Read the model definition and answer for the solid it produces. Units are mm, in the model's axes. A direction names the side the tool comes from. Coordinates: 2 decimals unless noted, no trailing zeros. Order: outer loops, then holes, each group sorted by start corner. A loop starts at its lowest first (then second) coordinate and runs counter-clockwise, first axis right, second up. Notation, with made-up numbers: (-39.5, 27.25) - (-23.5, 27.25) arc R21 ccw to (-23.5, 37.25) - close; hole circle Ø5 at (87.5, 31.25). An arc over 180 degrees is marked (long way). Answer as a JSON object with one key per item and string values. Group by question number.
from build123d import *

# Parameters (mm, degrees)
SKETCH1_W           = 12
SKETCH1_H           = 22
BOSS_EXTRUDE1_DEPTH = 23
SKETCH3_W           = 12
SKETCH3_H           = 2
BOSS_EXTRUDE3_DEPTH = 5
SKETCH2_R           = 6
BOSS_EXTRUDE4_DEPTH = 4
SKETCH4_R           = 2.5
BOSS_EXTRUDE5_DEPTH = 3


with BuildPart() as part:
    # Sketch1 → Boss-Extrude1 (new body)
    with BuildSketch(Plane(origin=(0, 0, 0), x_dir=(1, 0, 0), z_dir=(0, 1, 0))):
        Rectangle(SKETCH1_W, SKETCH1_H)
    extrude(amount=BOSS_EXTRUDE1_DEPTH)

    # Sketch3 → Boss-Extrude3 (add)
    with BuildSketch(Plane(origin=(0, 0, -11), x_dir=(-1, 0, 0), z_dir=(0, 0, -1))):
        with Locations((0, 18)):
            Rectangle(SKETCH3_W, SKETCH3_H)
    boss_extrude3 = extrude(amount=BOSS_EXTRUDE3_DEPTH)

    # Mirror1: Boss-Extrude3 across plane
    add(boss_extrude3.mirror(Plane.XY))

    # Sketch2 → Boss-Extrude4 (add)
    with BuildSketch(Plane(origin=(0, 23, 0), x_dir=(1, 0, 0), z_dir=(0, 1, 0))):
        with Locations(Location((0, -5, 0), (0, 0, 270))):
            Circle(SKETCH2_R)
    extrude(amount=BOSS_EXTRUDE4_DEPTH)

    # Sketch4 → Boss-Extrude5 (add)
    with BuildSketch(Plane(origin=(0, 27, 0), x_dir=(1, 0, 0), z_dir=(0, 1, 0))):
        with Locations(Location((0, -5, 0), (0, 0, 270))):
            Circle(SKETCH4_R)
    extrude(amount=BOSS_EXTRUDE5_DEPTH)


solid = part.part
1. A cutting plane is placed at B-B on y = 11.75. Write down the section's boundary in (x, z).
2. A cutting plane is placed at A-A on x = 4.75. Write down the section's boundary in (y, z), and give its area (3 significant figures).
3. For faces 1 (the flat face through (-5, 23, 10)), 2 (the flat face through (0, 21, 11)), 3 (the flat face through (0, 19, -13)), 4 (the flat face through (-3, 27, 5)), 5 (the flat face through (0, 8, -11)), determine the directions among +Z, -Z, +X, -X, +Y, -Y from which every point of the face is accessible in a straight line to the end or side of a thin tool.
4. A cutting plane is placed at D-D on x = -4. Write down the section's boundary in (y, z), and give its area (3 significant figures).
5. Straight lines are drawn through the part: L1, parallel to Z at x = 0.5, y = 21.25; L2, parallel to Y at x = -0.75, z = -9.5; L3, parallel to Y at x = -1, z = 10.5. For each, find the intervals that lie inside material, in ascending order.
6. Given pin 1 (1.8 mm diameter, centred on x = 3.5, z = 9, fed in from +Y); pin 2 (4 mm diameter, centred on x = -0.5, z = -13.5, fed in from -Y); pin 3 (2.5 mm diameter, centred on x = 2, z = -13.5, fed in from +Y), each flat-ended and moving along its own axis, determine where each tip first touches the part or whether it passes through.
7. A cutting plane is placed at C-C on z = 3.5. Write down the section's boundary in (x, y), and give its area (3 significant figures).
Derived:
{
 "1": {"outline": "(-6, -11) - (6, -11) - (6, 11) - (-6, 11) - close"},
 "2": {"outline": "(0, -11) - (17, -11) - (17, -16) - (19, -16) - (19, -11) - (23, -11) - (23, 1.33) - (27, 1.33) - (27, 8.67) - (23, 8.67) - (23, 11) - (19, 11) - (19, 16) - (17, 16) - (17, 11) - (0, 11) - close", "area": "555 mm2"},
 "3": {"face 1": "+Z, -X, +Y", "face 2": "+Z, +X, -X, +Y", "face 3": "-Z, +X, -X, +Y", "face 4": "+Y", "face 5": "-Z, +X, -X, -Y"},
 "4": {"outline": "(0, -11) - (17, -11) - (17, -16) - (19, -16) - (19, -11) - (23, -11) - (23, 0.53) - (27, 0.53) - (27, 9.47) - (23, 9.47) - (23, 11) - (19, 11) - (19, 16) - (17, 16) - (17, 11) - (0, 11) - close", "area": "562 mm2"},
 "5": {"L1": "z = -11 to 11", "L2": "y = 0 to 23", "L3": "y = 0 to 27"},
 "6": {"pin 1": "stops at y = 27", "pin 2": "stops at y = 17", "pin 3": "stops at y = 19"},
 "7": {"outline": "(-6, 0) - (6, 0) - (6, 23) - (5.81, 23) - (5.81, 27) - (2, 27) - (2, 30) - (-2, 30) - (-2, 27) - (-5.81, 27) - (-5.81, 23) - (-6, 23) - close", "area": "334 mm2"}
}
